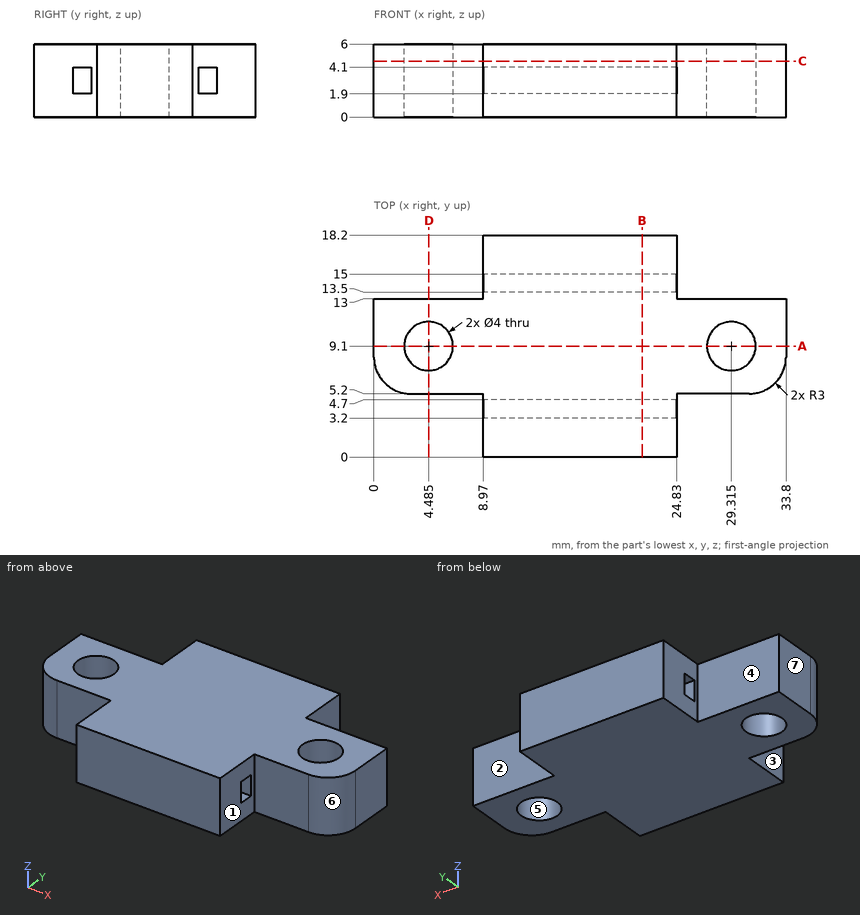
The figure shows three views and two pictorial views of one solid part (mm, origin at its lowest corner). Answer the questions. A direction names the side the tool comes from. Coordinates: 2 decimals unless noted, no trailing zeros. Write each loop counter-clockwise with the first axis right and the second up, starting at its lowest first coordinate (ties: lowest second). Pieces come first, ordered by that corner, then holes. Notation, with made-up numbers: M 24,-34.75 L 78,-34.75 A31 cw 78,-3.75 Z; hole C 64.25,36.25 d10. An arc over 180 degrees is marked long. Answer as CSV lines item,"result". Start each with the question number.
Item 1: Consider L1, parallel to Y at x = 23.5, z = 3.6; L2, parallel to Z at x = 13.5, y = 14.25; L3, parallel to X at y = 17.75, z = 2.2. Determine where each line is inside the solid, lowest interval first.
Item 2: Section A-A on y = 9.1 is taken. Write down the section's boundary in (x, z) (3 decimals), and give its area (3 significant figures).
Item 3: Determine the mould class of the marked faces 5, 6 and 7 for opening direction X: released by +X, released by -X, zero draft, split by the parting line, or undercut.
Item 4: A tool of negligible diameter and unlimited length cuts with its end or side. For the marked faces 1, 2, 3 and 4, from which of +Z, -Z, +X, -X, +Y, -Y can it reach the whole face along a straight path? Write none if from no direction.
Item 5: Section D-D on x = 4.5 is taken. Write down the section's boundary in (y, z).
Item 6: Flat-ended cylindrical pins translate along their axes: P1, Ø3, axis at x = 4.485, y = 9.1, coming from the -Z side; P2, Ø3, axis at x = 27.5, z = 2, coming from the +Y side; P3, Ø3, axis at x = 5.5, z = 3, coming from the -Y side. Find the tip coordinate at first contact, or state that the pin passes through.
Item 7: Section B-B on x = 22 is taken. Write down the section's boundary in (y, z).
Item 8: Section C-C on z = 4.6 is taken. Write down the section's boundary in (x, y) (3 decimals).
Checks:
1,L1,"y = 0 to 3.2, 4.7 to 13.5, 15 to 18.2"
1,L2,"z = 0 to 1.9, 4.1 to 6"
1,L3,"x = 8.97 to 24.83"
2,outline,"M 0,0 L 2.485,0 L 2.485,6 L 0,6 Z; M 6.485,0 L 27.315,0 L 27.315,6 L 6.485,6 Z; M 31.315,0 L 33.8,0 L 33.8,6 L 31.315,6 Z"
2,area,"155 mm²"
3,face 5,"undercut"
3,face 6,"released by +X"
3,face 7,"released by -X"
4,face 1,"+Z, -Z, +X, -Y"
4,face 2,"+Z, -Z, +X, +Y"
4,face 3,"+Z, -Z, -X, -Y"
4,face 4,"+Z, -Z, -X, +Y"
5,outline,"M 5.2,0 L 7.1,0 L 7.1,6 L 5.2,6 Z; M 11.1,0 L 13,0 L 13,6 L 11.1,6 Z"
6,P1,"passes through"
6,P2,"stops at y = 13"
6,P3,"stops at y = 5.2"
7,outline,"M 0,0 L 18.2,0 L 18.2,6 L 0,6 Z; hole M 3.2,1.9 L 4.7,1.9 L 4.7,4.1 L 3.2,4.1 Z; hole M 13.5,1.9 L 15,1.9 L 15,4.1 L 13.5,4.1 Z"
8,outline,"M 0,8.2 A3 ccw 3,5.2 L 8.97,5.2 L 8.97,0 L 24.83,0 L 24.83,5.2 L 30.8,5.2 A3 ccw 33.8,8.2 L 33.8,13 L 24.83,13 L 24.83,18.2 L 8.97,18.2 L 8.97,13 L 0,13 Z; hole C 4.485,9.1 d4; hole C 29.315,9.1 d4"
